The listing builds one solid part. Answer for the finished solid, in the listing's coordinates (mm). Coordinates: 2 decimals unless noted, no trailing zeros. Write each loop counter-clockwise with the first axis right and the second up, starting at its lowest first coordinate (ties: lowest second). Pieces come first, ordered by that corner, then holes. Notation, with made-up numbers: M 45,82 L 69,82 A4 ccw 69,87 Z; hole C 68,78.5 d6. An arc over 180 degrees is marked long. Answer as CSV lines item,"result".
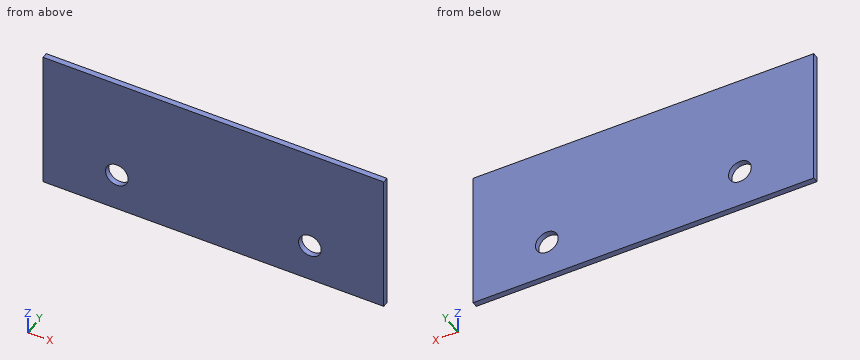
```python
from build123d import *

# Parameters (mm, degrees)
F0_W     = 1143
F0_H     = 469.9
F1_DEPTH = 19.05
F2_R     = 38.1
F3_DEPTH = 19.051


with BuildPart() as f1:
    # F0 (on Front) → F1 (new body)
    with BuildSketch(Plane.XZ):
        Rectangle(F0_W, F0_H)
    extrude(amount=F1_DEPTH)

    # F2 (on face) → F3 (cut, through all)
    with BuildSketch(Plane(origin=(0, 0, 0), x_dir=(-1, 0, 0), z_dir=(0, 1, 0))):
        with Locations((-323.85, -107.95)):
            Circle(F2_R)
        with Locations((323.85, -107.95)):
            Circle(F2_R)
    extrude(amount=-F3_DEPTH, mode=Mode.SUBTRACT)


solid = f1.part
```
Q1. Straight lines are drawn through the part: line 1 (Z direction, x = -323.85, y = -7.75); line 2 (X direction, y = -5, z = -118); line 3 (X direction, y = -1, z = -80). For each, find the intervals that lie inside material, in ascending order.
Output:
line 1,"-234.95 to -146.05, -69.85 to 234.95"
line 2,"-571.5 to -360.6, -287.1 to 287.1, 360.6 to 571.5"
line 3,"-571.5 to -349.74, -297.96 to 297.96, 349.74 to 571.5"
Q2. Find section A-A (z = -107.95). Give the vertices of the cut face in (x, y).
Output:
outline,"M -571.5,-19.05 L -361.95,-19.05 L -361.95,0 L -571.5,0 Z; M -285.75,-19.05 L 285.75,-19.05 L 285.75,0 L -285.75,0 Z; M 361.95,-19.05 L 571.5,-19.05 L 571.5,0 L 361.95,0 Z"
Q3. Find section C-C (y = -5.5). Give the vertices of the cut face in (x, z).
Output:
outline,"M -571.5,-234.95 L 571.5,-234.95 L 571.5,234.95 L -571.5,234.95 Z; hole C -323.85,-107.95 d76.2; hole C 323.85,-107.95 d76.2"
Q4. Find section B-B (x = -323.85). Give the vertices of the cut face in (y, z).
Output:
outline,"M -19.05,-234.95 L 0,-234.95 L 0,-146.05 L -19.05,-146.05 Z; M -19.05,-69.85 L 0,-69.85 L 0,234.95 L -19.05,234.95 Z"
